Check sheet for the modelled part. Datum: model origin and axes. Units: mm. Round coordinates to 2 decimals unless told otherwise and drop trailing zeros. Write each loop counter-clockwise with the first axis right and the second up, starting at its lowest first coordinate (ties: lowest second). Pieces come first, ordered by that corner, then holes. Notation, with made-up numbers: M 60,63 L 115,63 A17 ccw 115,78 Z; hole C 77.5,7 d7. An arc over 180 degrees is marked long. One line per item, written item: value.
from build123d import *

# Parameters (mm, degrees)
SKETCH_1_W          = 68
SKETCH_1_H          = 68
SKETCH_1_R          = 20
EXTRUDE_1_DEPTH     = 4
SKETCH_2_W          = 12
SKETCH_2_H          = 4
SKETCH_2_W_2        = 4
SKETCH_2_H_2        = 12
EXTRUDE_2_DEPTH     = 4
SKETCH_3_R          = 1.5
CUT_EXTRUDE_1_DEPTH = 4
FILLET_1_R          = 3
SKETCH_4_R          = 1.6
CUT_EXTRUDE_2_DEPTH = 10
SKETCH_5_R          = 2.1
CUT_EXTRUDE_3_DEPTH = 5


with BuildPart() as part:
    # 草图1 → 凸台-拉伸1 (new body)
    with BuildSketch(Plane(origin=(0, 0, 0), x_dir=(1, 0, 0), z_dir=(0, 1, 0))):
        Rectangle(SKETCH_1_W, SKETCH_1_H)
        with Locations(Location((0, 0, 0), (0, 0, 270))):
            Circle(SKETCH_1_R, mode=Mode.SUBTRACT)
    extrude(amount=EXTRUDE_1_DEPTH)

    # 草图2 → 凸台-拉伸2 (add)
    with BuildSketch(Plane(origin=(0, 4, 0), x_dir=(1, 0, 0), z_dir=(0, 1, 0))):
        with Locations((-15, 36)):
            Rectangle(SKETCH_2_W, SKETCH_2_H)
        with Locations((15, 36)):
            Rectangle(SKETCH_2_W, SKETCH_2_H)
        with Locations((36, 15)):
            Rectangle(SKETCH_2_W_2, SKETCH_2_H_2)
        with Locations((36, -15)):
            Rectangle(SKETCH_2_W_2, SKETCH_2_H_2)
        with Locations((15, -36)):
            Rectangle(SKETCH_2_W, SKETCH_2_H)
        with Locations((-15, -36)):
            Rectangle(SKETCH_2_W, SKETCH_2_H)
        with Locations((-36, -15)):
            Rectangle(SKETCH_2_W_2, SKETCH_2_H_2)
        with Locations((-36, 15)):
            Rectangle(SKETCH_2_W_2, SKETCH_2_H_2)
    extrude(amount=-EXTRUDE_2_DEPTH)

    # 草图3 → 切除-拉伸1 (cut)
    with BuildSketch(Plane(origin=(0, 4, 0), x_dir=(1, 0, 0), z_dir=(0, 1, 0))):
        with Locations((-22.5, 34)):
            Circle(SKETCH_3_R)
        with Locations((-7.5, 34)):
            Circle(SKETCH_3_R)
        with Locations((7.5, 34)):
            Circle(SKETCH_3_R)
        with Locations((22.5, 34)):
            Circle(SKETCH_3_R)
        with Locations((34, 22.5)):
            Circle(SKETCH_3_R)
        with Locations((34, 7.5)):
            Circle(SKETCH_3_R)
        with Locations((34, -7.5)):
            Circle(SKETCH_3_R)
        with Locations((34, -22.5)):
            Circle(SKETCH_3_R)
        with Locations((22.5, -34)):
            Circle(SKETCH_3_R)
        with Locations((7.5, -34)):
            Circle(SKETCH_3_R)
        with Locations((-7.5, -34)):
            Circle(SKETCH_3_R)
        with Locations((-22.5, -34)):
            Circle(SKETCH_3_R)
        with Locations((-34, -22.5)):
            Circle(SKETCH_3_R)
        with Locations((-34, -7.5)):
            Circle(SKETCH_3_R)
        with Locations((-34, 7.5)):
            Circle(SKETCH_3_R)
        with Locations((-34, 22.5)):
            Circle(SKETCH_3_R)
    extrude(amount=-CUT_EXTRUDE_1_DEPTH, mode=Mode.SUBTRACT)

    # 圆角1
    fillet_1_edges = [part.edges().sort_by_distance(p)[0] for p in [
        (34, 2, 34),
        (-34, 2, 34),
        (-34, 2, -34),
        (34, 2, -34),
    ]]
    fillet(fillet_1_edges, radius=FILLET_1_R)

    # 草图4 → 切除-拉伸2 (cut)
    with BuildSketch(Plane(origin=(0, 4, 0), x_dir=(1, 0, 0), z_dir=(0, 1, 0))):
        with Locations(Location((25, 0, 0), (0, 0, 270))):
            Circle(SKETCH_4_R)
        with Locations(Location((12.5, -21.650635095, 0), (0, 0, 270))):
            Circle(SKETCH_4_R)
        with Locations(Location((-12.5, -21.650635095, 0), (0, 0, 270))):
            Circle(SKETCH_4_R)
        with Locations(Location((-25, 0, 0), (0, 0, 270))):
            Circle(SKETCH_4_R)
        with Locations(Location((-12.5, 21.650635095, 0), (0, 0, 270))):
            Circle(SKETCH_4_R)
        with Locations(Location((12.5, 21.650635095, 0), (0, 0, 270))):
            Circle(SKETCH_4_R)
    extrude(amount=-CUT_EXTRUDE_2_DEPTH, mode=Mode.SUBTRACT)

    # 草图5 → 切除-拉伸3 (cut)
    with BuildSketch(Plane(origin=(0, 4, 0), x_dir=(1, 0, 0), z_dir=(0, 1, 0))):
        with Locations(Location((23.68807717, 23.68807717, 0), (0, 0, 270))):
            Circle(SKETCH_5_R)
        with Locations(Location((23.68807717, -23.68807717, 0), (0, 0, 270))):
            Circle(SKETCH_5_R)
        with Locations(Location((-23.68807717, -23.68807717, 0), (0, 0, 270))):
            Circle(SKETCH_5_R)
        with Locations(Location((-23.68807717, 23.68807717, 0), (0, 0, 270))):
            Circle(SKETCH_5_R)
    extrude(amount=-CUT_EXTRUDE_3_DEPTH, mode=Mode.SUBTRACT)


solid = part.part
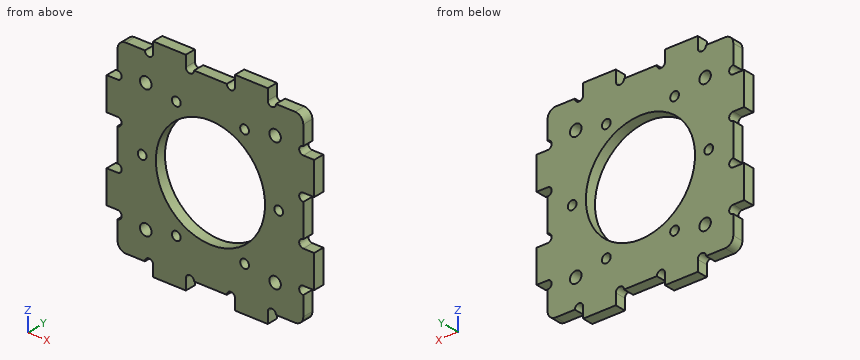
Q1. Scan lines: line 1 (X direction, y = 2.15, z = 0); line 2 (X direction, y = 0.85, z = -25.5); line 3 (X direction, y = 0.85, z = -25). Record each from-to range of solid material in increasing order. Write a range as [from, to].
Completed:
line 1: [-34, -26.6], [-23.4, -20], [20, 23.4], [26.6, 34]
line 2: [-34, -24.75], [-22.63, 22.63], [24.75, 34]
line 3: [-34, -25.33], [-22.05, 22.05], [25.33, 34]
Q2. Depth check by flat-ended pin: P1, Ø2, axis at y = 0.5, z = -2.5, coming from the -X side; P2, Ø1.2, axis at x = 37, y = 1.5, coming from the +Z side; P3, Ø2, axis at y = 1.5, z = -3, coming from the +X side; P4, Ø3, axis at x = 12.5, z = 21.65, coming from the +Y side. Enter the tip coordinate at first touch or a pass-through.
Completed:
P1: x = -34
P2: z = 21
P3: x = 34
P4: through
Q3. Sectioned sample at D-D on z = -8. Enter the section's corners in (x, y), and give its area (3 significant figures).
Completed:
outline: M -32.59,0 L -18.33,0 L -18.33,4 L -32.59,4 Z; M 18.33,0 L 32.59,0 L 32.59,4 L 18.33,4 Z
area: 114 mm^2
Q4. Sectioned sample at B-B on z = 0. Enter the section's corners in (x, y).
Completed:
outline: M -34,0 L -26.6,0 L -26.6,4 L -34,4 Z; M -23.4,0 L -20,0 L -20,4 L -23.4,4 Z; M 20,0 L 23.4,0 L 23.4,4 L 20,4 Z; M 26.6,0 L 34,0 L 34,4 L 26.6,4 Z
Q5. Sectioned sample at C-C on x = -22.5. Enter the section's corners in (y, z), and give its area (3 significant figures).
Completed:
outline: M 0,-32.5 L 4,-32.5 L 4,-25.42 L 0,-25.42 Z; M 0,-21.96 L 4,-21.96 L 4,21.96 L 0,21.96 Z; M 0,25.42 L 4,25.42 L 4,32.5 L 0,32.5 Z
area: 232 mm^2
Q6. Sectioned sample at A-A on x = 0. Enter the section's corners in (y, z).
Completed:
outline: M 0,-34 L 4,-34 L 4,-20 L 0,-20 Z; M 0,20 L 4,20 L 4,34 L 0,34 Z
